CAD build for the part. Positions are in the model's coordinates, mm. A direction names the side the tool comes from. Coordinates: 2 decimals unless noted, no trailing zeros. Loops run counter-clockwise (first coordinate to the right, second up) from the corner with the lowest first, then second, coordinate; pieces in that order, holes last. Notation, with made-up numbers: (-8, 60) -> (15, 60) arc R26 ccw to (15, 76) -> close; hole circle Ø8 at (-27, 19). An arc over 180 degrees is marked (long way). Answer as CSV lines item,"result". Start each with the question number.
Autodesk Inventor part; units mm, degrees
ref_plane "YZ Plane" through (0, 0, 0) normal (1, 0, 0) x (0, 1, 0)
ref_plane "XZ Plane" through (0, 0, 0) normal (0, 1, 0) x (-1, 0, 0)
ref_plane "XY Plane" through (0, 0, 0) normal (0, 0, 1) x (1, 0, 0)
sketch "Sketch1" plane through (0, 0, 0) normal (0, 0, 1) x (1, 0, 0)
  line L0 (-25.4, 15.1328) -> (31.75, 15.1328)
  line L1 (31.75, 15.1328) -> (31.75, -22.9672)
  line L2 (31.75, -22.9672) -> (-25.4, -22.9672)
  line L3 (-25.4, -22.9672) -> (-25.4, 15.1328)
  point P0 (0, 0)
  dimension "d0" = 57.15
  dimension "d1" = 38.1
extrude "Extrusion1" add sketch "Sketch1" along normal blind 25.4
sketch "Sketch2" plane through (0, 0, 25.4) normal (0, 0, 1) x (1, 0, 0)
  line L0 (-25.4, 15.1328) -> (-25.4, -22.9672)
  line L1 (31.75, 15.1328) -> (-25.4, 15.1328)
  line L2 (-25.4, -3.9172) -> (0, -3.9172)
  line L3 (0, -3.9172) -> (0, 15.1328)
  line L4 (0, 15.1328) -> (-25.4, 15.1328)
  line L5 (-25.4, 15.1328) -> (-25.4, -3.9172)
  point P0 (0, 0)
  dimension "d4" = 19.05
  dimension "d5" = 25.4
extrude "Extrusion2" cut sketch "Sketch2" against normal blind 12.7
sketch "Sketch3" plane through (31.75, -22.9672, 0) normal (1, 0, 0) x (0, 0, -1)
  line L0 (0, 0) -> (-25.4, 0)
  line L1 (0, 38.1) -> (-25.4, 38.1)
  line L2 (-12.7, 0) -> (-25.4, 0)
  line L3 (-25.4, 0) -> (-25.4, 38.1)
  line L4 (-25.4, 38.1) -> (-12.7, 38.1)
  line L5 (-12.7, 38.1) -> (-12.7, 0)
  point P0 (0, 22.9672)
  dimension "d8" = 12.7
extrude "Extrusion3" cut sketch "Sketch3" against normal blind 12.7
properties part number "Figure 7_27_3"
Item 1: Saw through at A-A (y = 12). Write the cut outline in (x, z), plus the area to 3 significant figures.
Item 2: Saw through at D-D (x = 26). Write the cut outline in (y, z), plus the area to 3 significant figures.
Item 3: Saw through at B-B (x = -21). Write the cut outline in (y, z), plus the area to 3 significant figures.
Item 4: Saw through at C-C (z = 20). Write the cut outline in (x, y).
Item 5: Which spindle directions (+Z, -Z, +X, -X, +Y, -Y) get a long thin tool onto all of the face, cutting with end or side? Do faces 1 (the face through (31.75, -4, 6)), 2 (the face through (0, 5, 19)), 3 (the face through (19.05, -4, 19)). Say none if no direction does.
Item 6: Wall check: probe 1 along Y at (x, z) = (-21.5, 18.25); probe 2 along Z at (x, y) = (-21.5, 11); probe 3 along X at (y, z) = (12, 15.5). Give the ranges that are in metal, low to high.
Item 7: Flat gauge pins, fed straight in: pin 1 Ø6.5 at (y, z) = (-11, 16.5) entering from +X; pin 2 Ø4 at (x, z) = (-7, 21.5) entering from +Y; pin 3 Ø1 at (x, y) = (25.5, -17) entering from +Z. Where does each tip first touch, or does it go through?
Geometry check:
1,outline,"(-25.4, 0) -> (31.75, 0) -> (31.75, 12.7) -> (19.05, 12.7) -> (19.05, 25.4) -> (0, 25.4) -> (0, 12.7) -> (-25.4, 12.7) -> close"
1,area,"968 mm2"
2,outline,"(-22.97, 0) -> (15.13, 0) -> (15.13, 12.7) -> (-22.97, 12.7) -> close"
2,area,"484 mm2"
3,outline,"(-22.97, 0) -> (15.13, 0) -> (15.13, 12.7) -> (-3.92, 12.7) -> (-3.92, 25.4) -> (-22.97, 25.4) -> close"
3,area,"726 mm2"
4,outline,"(-25.4, -22.97) -> (19.05, -22.97) -> (19.05, 15.13) -> (0, 15.13) -> (0, -3.92) -> (-25.4, -3.92) -> close"
5,face 1,"+Z, -Z, +X, +Y, -Y"
5,face 2,"+Z, -X, +Y"
5,face 3,"+Z, +X, +Y, -Y"
6,probe 1,"-22.97 to -3.92"
6,probe 2,"0 to 12.7"
6,probe 3,"0 to 19.05"
7,pin 1,"x = 19.05"
7,pin 2,"y = -3.92"
7,pin 3,"z = 12.7"
